Read the model definition and answer for the solid it produces. Units are mm, in the model's axes. A direction names the side the tool comes from. Coordinates: 2 decimals unless noted, no trailing zeros. Write each loop counter-clockwise with the first axis right and the second up, starting at its lowest first coordinate (ties: lowest second). Pieces come first, ordered by that corner, then holes. Notation, with made-up numbers: (63, -21.75) -> (107, -21.75) arc R26 cw to (107, 13.25) -> close; hole circle Ø5 at (82, 71). An arc over 180 degrees is marked (long way). One line per item, written item: value. Start each with the question number.
from build123d import *

# Parameters (mm, degrees)
BOSS_EXTRUDE1_START     = -31
SKETCH1_W               = 19
SKETCH1_H               = 6
BOSS_EXTRUDE1_DEPTH     = 6
BOSS_EXTRUDE2_REACH     = 726.688
SKETCH2_W               = 38
SKETCH2_H               = 6
SKETCH3_R               = 1.5
CUT_EXTRUDE1_DEPTH      = 744.440196757
FILLET1_R               = 1
CUT_EXTRUDE3_DEPTH      = 744.257611618
CUT_EXTRUDE3_DEPTH_BACK = 744.257611618
SKETCH5_R               = 1.5
CUT_EXTRUDE4_DEPTH      = 744.257611618


with BuildPart() as part:
    # Sketch1 → Boss-Extrude1 (new body)
    with BuildSketch(Plane.XY.offset(BOSS_EXTRUDE1_START)):
        with Locations((714.5, 128)):
            Rectangle(SKETCH1_W, SKETCH1_H)
    extrude(amount=BOSS_EXTRUDE1_DEPTH)

    # Boss-Extrude2: up to this plane
    boss_extrude2_end = Plane(origin=(203.909377292, 470.655270204, 323.5), z_dir=(-0.5307002791731883, -0.8475595635030614, 0))
    # Sketch2 → Boss-Extrude2 (add, up to the surface)
    with BuildSketch(Plane(origin=(0, 131, 0), x_dir=(1, 0, 0), z_dir=(0, 1, 0)), mode=Mode.PRIVATE) as boss_extrude2_sk1:
        with Locations((705, 28)):
            Rectangle(SKETCH2_W, SKETCH2_H)
    boss_extrude2_tool1 = split(extrude(boss_extrude2_sk1.sketch, amount=BOSS_EXTRUDE2_REACH, mode=Mode.PRIVATE), bisect_by=boss_extrude2_end, keep=Keep.BOTH, mode=Mode.PRIVATE)
    add(boss_extrude2_tool1.solids().sort_by_distance((705, 131, -28))[0])

    # Sketch3 → Cut-Extrude1 (cut, through all)
    with BuildSketch(Plane.XY.offset(-25)):
        with Locations((705, 131)):
            Circle(SKETCH3_R)
    extrude(amount=-CUT_EXTRUDE1_DEPTH, mode=Mode.SUBTRACT)

    # Fillet1
    fillet1_edges = [part.edges().sort_by_distance(p)[0] for p in [
        (686, 168.79373849, -28),
    ]]
    fillet(fillet1_edges, radius=FILLET1_R)

    # Sketch4 → Cut-Extrude3 (cut, two sides: drawn at the far end of the back side and taken through both)
    with BuildSketch(Plane.XY.offset(-25).offset(-CUT_EXTRUDE3_DEPTH_BACK)):
        Polygon((701.75741477, 158.927217271), (698.573213095, 153.84185989), (724, 137.920851515), (727.184201675, 143.006208896), align=None)
    extrude(amount=CUT_EXTRUDE3_DEPTH + CUT_EXTRUDE3_DEPTH_BACK, mode=Mode.SUBTRACT)

    # Sketch5 → Cut-Extrude4 (cut, through all)
    with BuildSketch(Plane.XY.offset(-25)):
        with Locations((698.573213095, 153.84185989)):
            Circle(SKETCH5_R)
    extrude(amount=-CUT_EXTRUDE4_DEPTH, mode=Mode.SUBTRACT)


solid = part.part
1. A cutting plane is placed at C-C on x = 695. Give the vertices of the cut face in (y, z).
2. A cutting plane is placed at B-B on y = 154. Give the vertices of the cut face in (x, z), then the cut area to 3 significant figures.
3. Find the intervals of material crossed by probe 1 along X at (y, z) = (154, -25.25); probe 2 along Y at (x, z) = (688.5, -28.5); probe 3 along X at (y, z) = (143, -26), in increasing order. Write a range as from..to.
4. A cutting plane is placed at A-A on z = -25.5. Give the vertices of the cut face in (x, y).
5. A tool of negligible diameter and unlimited length cuts with its end or side. For faces 5 (the face through (701, 141, -25)), 6 (the face through (695, 131, -28)), from which of +Z, -Z, +X, -X, +Y, -Y can it reach the whole face along a straight path? Write none if from no direction.
6. Given pin 1 (3 mm diameter, centred on x = 695.5, z = -28, fed in from -Y); pin 2 (3 mm diameter, centred on x = 706, z = -29, fed in from +Y); pin 3 (1 mm diameter, centred on x = 696.5, z = -26, fed in from +Y), each flat-ended and moving along its own axis, determine where each tip first touches the part or whether it passes through.
7. For a pull along Y with two mould halves and no side action, classify faces 1 (the face through (701, 141, -31)), 2 (the face through (714, 125, -28)), 3 (the face through (700.58, 157.05, -28.04)), 4 (the face through (686.503, 167.855, -27.958)) as +Y half, -Y half, draft (parallel to the pull), parting line (faces both ways), or undercut.
Derived:
1. outline: (131, -31) -> (163.16, -31) -> (163.16, -25) -> (131, -25) -> close
2. outline: (686, -31) -> (697.08, -31) -> (697.08, -25) -> (686, -25) -> close
2. area: 66.5 mm2
3. probe 1: x = 686..697.08
3. probe 2: y = 131..167.23
3. probe 3: x = 686..715.89
4. outline: (686, 131) -> (703.5, 131) arc R1.5 cw (long way) to (705, 129.5) -> (705, 125) -> (724, 125) -> (724, 137.92) -> (699.84, 153.05) arc R1.5 cw (long way) to (699.37, 155.11) -> (701.76, 158.93) -> (687.53, 167.84) arc R1 ccw to (686, 166.99) -> close
5. face 5: +Z, +X, -X, +Y, -Y
5. face 6: +Z, -Z, -X, -Y
6. pin 1: stops at y = 131
6. pin 2: stops at y = 150.13
6. pin 3: stops at y = 162.53
7. face 1: draft
7. face 2: -Y half
7. face 3: undercut
7. face 4: +Y half
